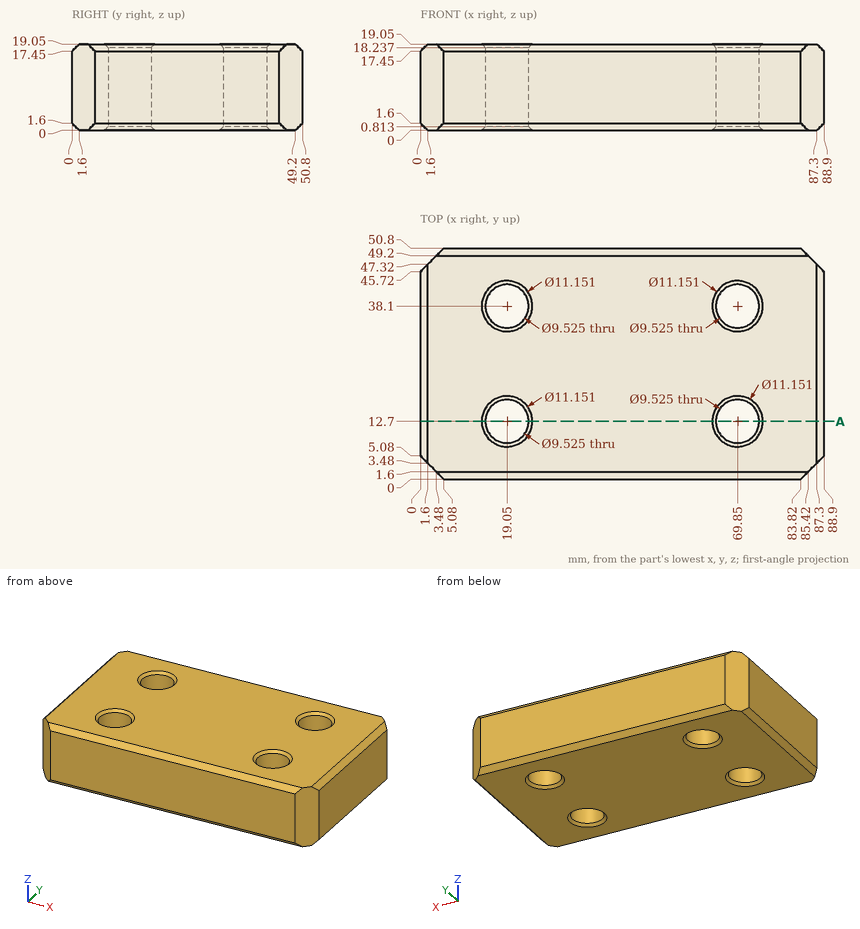
Geometry check sheet. Reference: drawing and pictorial views, mm from the part's lowest x, y, z. Coordinates: 2 decimals unless noted, no trailing zeros.
Item 1: Scan lines: line 1 along Y through (x, z) = (69.85, 6.5); line 2 along X through (y, z) = (35.5, 5.5); line 3 along X through (y, z) = (11, 5.25). Record each from-to range of solid material in increasing order.
Item 2: Section check A-A (y = 12.7). Count the separate pieces of the cut face and the enclosed holes in it, plus the area to 3 significant figures.
Item 3: Depth check by flat-ended pin: pin 1 (5.5 mm diameter, centred on x = 69.85, y = 38.1, fed in from -Z); pin 2 (11 mm diameter, centred on x = 69.85, y = 12.7, fed in from +Z) (1 decimal). Enter the tip coordinate at first touch or a pass-through.
Check sheet entries:
1. line 1: y = 0 to 7.94, 17.46 to 33.34, 42.86 to 50.8
1. line 2: x = 0 to 15.06, 23.04 to 65.86, 73.84 to 88.9
1. line 3: x = 0 to 14.6, 23.5 to 65.4, 74.3 to 88.9
2. separate pieces: 3
2. enclosed holes: 0
2. area: 1,320 mm2
3. pin 1: passes through
3. pin 2: stops at z = 19
